Design review of the part built by this model. Coordinates are the model's own, in mm. Face numbers are marked on the shaded views. Coordinates: 2 decimals unless noted, no trailing zeros. Order: outer loops, then holes, each group sorted by start corner. A loop starts at its lowest first (then second) coordinate and runs counter-clockwise, first axis right, second up. Notation, with made-up numbers: M -24.75,13 L -17.75,13 A30 cw -17.75,52 Z; hole C -28.5,38 d8. An arc over 180 degrees is marked long. Answer as a JSON object with one key per item and string values.
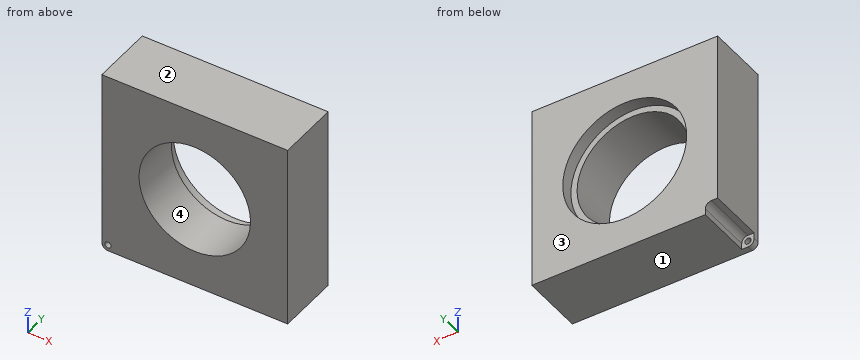
from build123d import *

# Parameters (mm, degrees)
SKETCH1_W           = 150
SKETCH1_H           = 150
BOSS_EXTRUDE1_DEPTH = 50
SKETCH2_R           = 50
CUT_EXTRUDE1_DEPTH  = 10
SKETCH3_R           = 45
CUT_EXTRUDE2_DEPTH  = 114.357840488
SKETCH4_W           = 10
SKETCH4_H           = 10
CUT_EXTRUDE3_DEPTH  = 45
SKETCH6_R           = 2.55
CUT_EXTRUDE4_DEPTH  = 5
FILLET1_R           = 5


with BuildPart() as part:
    # Sketch1 → Boss-Extrude1 (new body)
    with BuildSketch(Plane(origin=(0, 0, 0), x_dir=(1, 0, 0), z_dir=(0, 1, 0))):
        Rectangle(SKETCH1_W, SKETCH1_H)
    extrude(amount=BOSS_EXTRUDE1_DEPTH)

    # Sketch2 → Cut-Extrude1 (cut)
    with BuildSketch(Plane(origin=(0, 50, 0), x_dir=(1, 0, 0), z_dir=(0, 1, 0))):
        with Locations(Location((0, 0, 0), (0, 0, 270))):
            Circle(SKETCH2_R)
    extrude(amount=-CUT_EXTRUDE1_DEPTH, mode=Mode.SUBTRACT)

    # Sketch3 → Cut-Extrude2 (cut, through all)
    with BuildSketch(Plane(origin=(0, 40, 0), x_dir=(1, 0, 0), z_dir=(0, 1, 0))):
        with Locations(Location((0, 0, 0), (0, 0, 270))):
            Circle(SKETCH3_R)
    extrude(amount=-CUT_EXTRUDE2_DEPTH, mode=Mode.SUBTRACT)

    # Sketch4 → Cut-Extrude3 (cut)
    with BuildSketch(Plane(origin=(0, 50, 0), x_dir=(1, 0, 0), z_dir=(0, 1, 0))):
        with Locations((-70, 70)):
            Rectangle(SKETCH4_W, SKETCH4_H)
    extrude(amount=-CUT_EXTRUDE3_DEPTH, mode=Mode.SUBTRACT)

    # Sketch6 → Cut-Extrude4 (cut)
    with BuildSketch(Plane(origin=(0, 5, 0), x_dir=(1, 0, 0), z_dir=(0, 1, 0))):
        with Locations(Location((-70, 70, 0), (0, 0, 270))):
            Circle(SKETCH6_R)
    extrude(amount=-CUT_EXTRUDE4_DEPTH, mode=Mode.SUBTRACT)

    # Fillet1
    fillet1_edges = [part.edges().sort_by_distance(p)[0] for p in [
        (-75, 2.5, -75),
        (-65, 27.5, -65),
    ]]
    fillet(fillet1_edges, radius=FILLET1_R)


solid = part.part
1) To check wall thickness, follow L1, parallel to X at y = 9, z = 0; L2, parallel to Z at x = 15, y = 38; L3, parallel to Z at x = 6, y = 11. State the ranges of each line that lie inside material, in increasing order.
Taken from the geometry:
{"L1": "x = -75 to -45, 45 to 75", "L2": "z = -75 to -42.43, 42.43 to 75", "L3": "z = -75 to -44.6, 44.6 to 75"}
2) Add section D-D (y = 44). State the section outline as (x, z) points.
Taken from the geometry:
{"outline": "M -75,-65 L -70,-65 A5 cw -65,-70 L -65,-75 L 75,-75 L 75,75 L -75,75 Z; hole C 0,0 d100"}
3) Insertion check: pin 1 Ø5 at (x, z) = (-69.5, -71.5) entering from +Y; pin 2 Ø4 at (y, z) = (18, -72.5) entering from -X; pin 3 Ø5.5 at (x, y) = (-72.5, 37.5) entering from -Z; pin 4 Ø10 at (x, z) = (-14, 42) entering from -Y. Each pin has a flat end and moves straight along its axis. Give the tip position at first contact, or say it passes through.
Taken from the geometry:
{"pin 1": "stops at y = 5", "pin 2": "stops at x = -65", "pin 3": "stops at z = -65.01", "pin 4": "stops at y = 0"}
4) Mouldability with a two-part tool opening along Z and no side actions: class the marked faces 1, 2, 3 and 4 as released by +Z, released by -Z, zero draft, split by the parting line, or undercut.
Taken from the geometry:
{"face 1": "released by -Z", "face 2": "released by +Z", "face 3": "zero draft", "face 4": "undercut"}
5) Add section C-C (x = 5). State the section outline as (y, z) points.
Taken from the geometry:
{"outline": "M 0,-75 L 50,-75 L 50,-49.75 L 40,-49.75 L 40,-44.72 L 0,-44.72 Z; M 0,44.72 L 40,44.72 L 40,49.75 L 50,49.75 L 50,75 L 0,75 Z"}
6) Add section B-B (z = 0). State the section outline as (x, y) points.
Taken from the geometry:
{"outline": "M -75,0 L -45,0 L -45,40 L -50,40 L -50,50 L -75,50 Z; M 45,0 L 75,0 L 75,50 L 50,50 L 50,40 L 45,40 Z"}
7) Add section A-A (y = 32). State the section outline as (x, z) points.
Taken from the geometry:
{"outline": "M -75,-65 L -70,-65 A5 cw -65,-70 L -65,-75 L 75,-75 L 75,75 L -75,75 Z; hole C 0,0 d90"}
